Could you check a few things on this model? Use its own coordinates, in mm. Face numbers are marked on the shaded views. A direction names the side the tool comes from. Give positions to 0.01 mm unless a question says otherwise; leave off trailing zeros. Order: outer loops, then holes, each group sorted by start corner. A loop starts at its lowest first (then second) coordinate and runs counter-clockwise, first axis right, second up. Notation, with made-up numbers: M 73,23.5 L 114,23.5 A13 ccw 114,32.5 Z; hole C 55,72.5 d10. An arc over 180 degrees is marked long. Use a Markdown table: item, result. Add a question column.
```python
from build123d import *

# Parameters (mm, degrees)
BOSS_EXTRUDE1_DEPTH      = 50.8
BOSS_EXTRUDE1_DEPTH_BACK = 8.89
SKETCH3_W                = 168.91
SKETCH3_H                = 143.51
SKETCH3_W_2              = 148.59
SKETCH3_H_2              = 123.19
SKETCH3_3_W              = 148.59
SKETCH3_3_H              = 123.19
BOSS_EXTRUDE2_DEPTH      = 8.89
BOSS_EXTRUDE3_DEPTH      = 59.69
CUT_EXTRUDE1_DEPTH       = 239.691156361
CUT_EXTRUDE1_DEPTH_BACK  = 239.691156361
SKETCH5_R                = 4.445
SKETCH5_R_2              = 1.000000032
SKETCH5_R_3              = 1
FILLET1_R                = 5.08
SKETCH7_W                = 88.9
SKETCH7_H                = 95.25
BOSS_EXTRUDE4_DEPTH      = 12.7
CHAMFER1_SIZE            = 21.336
CHAMFER2_START           = -153
CHAMFER2_OUTLINE_W       = 18
CHAMFER2_OUTLINE_H       = 17
CHAMFER2_DEPTH           = 6.894626535
CHAMFER3_START           = -186
CHAMFER3_OUTLINE_W       = 15
CHAMFER3_OUTLINE_H       = 17
CHAMFER3_DEPTH           = 6.430939091
CHAMFER4_SIZE            = 5.08
CHAMFER5_SIZE            = 5.08
FILLET3_R                = 10.16
CHAMFER6_SIZE            = 5.08
CUT_EXTRUDE2_DEPTH       = 275.484237722
CUT_EXTRUDE2_DEPTH_BACK  = 275.484237722
SKETCH8_R                = 5.08
SKETCH9_R                = 2
SKETCH9_R_2              = 2.000000064
CUT_EXTRUDE3_DEPTH       = 12.7
SKETCH10_W               = 12.7
SKETCH10_H               = 43.18
BOSS_EXTRUDE5_DEPTH      = 50.8
SKETCH11_W               = 27.305
SKETCH11_H               = 50.8
CUT_EXTRUDE4_DEPTH       = 12.7
FILLET4_R                = 5.08
SKETCH12_R               = 15.875
CUT_EXTRUDE5_DEPTH       = 2.032
CUT_EXTRUDE6_START       = -2.032
SKETCH13_R               = 15.875
CUT_EXTRUDE6_DEPTH       = 2.032
FILLET5_R                = 5.08
FILLET6_R                = 5.08
SKETCH15_R               = 7.62
CUT_EXTRUDE7_DEPTH       = 5.08
BOSS_EXTRUDE6_DEPTH      = 12.7
FILLET9_R                = 6.35
BOSS_EXTRUDE7_START      = -12.7
BOSS_EXTRUDE7_DEPTH      = 12.7


with BuildPart() as part:
    # Sketch3 → Boss-Extrude1 (new, two sides: drawn at the far end of the back side and taken through both)
    with BuildSketch(Plane(origin=(0, 0, 0), x_dir=(1, 0, 0), z_dir=(0, 1, 0)).offset(-BOSS_EXTRUDE1_DEPTH_BACK)):
        Rectangle(SKETCH3_W, SKETCH3_H)
        Rectangle(SKETCH3_W_2, SKETCH3_H_2, mode=Mode.SUBTRACT)
    extrude(amount=BOSS_EXTRUDE1_DEPTH + BOSS_EXTRUDE1_DEPTH_BACK)

    # Sketch3<3> → Boss-Extrude2 (add)
    with BuildSketch(Plane(origin=(0, 0, 0), x_dir=(1, 0, 0), z_dir=(0, 1, 0))):
        Rectangle(SKETCH3_3_W, SKETCH3_3_H)
    extrude(amount=-BOSS_EXTRUDE2_DEPTH)

    # Sketch4 → Boss-Extrude3 (add)
    with BuildSketch(Plane(origin=(0, -8.89, 0), x_dir=(-1, 0, 0), z_dir=(0, -1, 0))):
        Polygon((137.454999918, 60.325), (84.455, 60.325), (84.455, 43.815), (126.024999918, 43.815), (126.024999918, 23.495), (137.454999918, 23.495), align=None)
        Polygon((126.025, -43.815), (84.455, -43.815), (84.455, -60.325), (137.455, -60.325), (137.455, -23.495), (126.025, -23.495), align=None)
        Polygon((-84.455, 43.815), (-84.455, 60.325), (-137.454999918, 60.325), (-137.454999918, 23.495), (-126.024999918, 23.495), (-126.024999918, 43.815), align=None)
        Polygon((-84.455, -43.815), (-126.025, -43.815), (-126.025, -23.495), (-137.455, -23.495), (-137.455, -60.325), (-84.455, -60.325), align=None)
    extrude(amount=-BOSS_EXTRUDE3_DEPTH)

    # Sketch5 → Cut-Extrude1 (cut, two sides: drawn at the far end of the back side and taken through both)
    with BuildSketch(Plane.ZY.offset(84.455).offset(-CUT_EXTRUDE1_DEPTH_BACK)):
        with Locations(Location((0, 20.955, 0), (0, 0, 180))):
            Circle(SKETCH5_R)
        with Locations(Location((-9.017, 20.955, 0), (0, 0, 180))):
            Circle(SKETCH5_R_2)
        with Locations(Location((9.017, 20.955, 0), (0, 0, 180))):
            Circle(SKETCH5_R_3)
        with Locations(Location((0.017538483, 29.972, 0), (0, 0, 180))):
            Circle(SKETCH5_R_3)
        with Locations(Location((-0.055629344, 11.938, 0), (0, 0, 180))):
            Circle(SKETCH5_R_3)
    extrude(amount=CUT_EXTRUDE1_DEPTH + CUT_EXTRUDE1_DEPTH_BACK, mode=Mode.SUBTRACT)

    # Fillet1
    fillet1_edges = [part.edges().sort_by_distance(p)[0] for p in [
        (84.455, 20.955, -60.325),
        (84.455, 20.955, -43.815),
        (-84.455, 20.955, -43.815),
        (-84.455, 20.955, -60.325),
        (-84.455, 20.955, 43.815),
        (-84.455, 20.955, 60.325),
        (84.455, 20.955, 71.755),
        (-84.455, 20.955, 71.755),
        (84.455, 20.955, 60.325),
        (84.455, 20.955, 43.815),
    ]]
    fillet(fillet1_edges, radius=FILLET1_R)

    # Sketch7 → Boss-Extrude4 (add)
    with BuildSketch(Plane.ZY.offset(84.455)):
        with Locations((-116.205, 28.287736962)):
            Rectangle(SKETCH7_W, SKETCH7_H)
    extrude(amount=-BOSS_EXTRUDE4_DEPTH)

    # Chamfer1
    # the kernel refuses this chamfer: 21.336 mm, written as the material it takes off along each edge
    with BuildSketch(Plane(origin=(-139.324428231, 75.912736962, -71.755), x_dir=(0, -1, 0), z_dir=(1, 0, 0))) as chamfer1_piece_1:
        Polygon((CHAMFER1_SIZE, 0), (0, CHAMFER1_SIZE), (0, 0), align=None)
    extrude(amount=122.438856462, mode=Mode.SUBTRACT)
    with BuildSketch(Plane(origin=(-139.324428231, -19.337263038, -71.755), x_dir=(0, 1, 0), z_dir=(1, 0, 0))) as chamfer1_piece_2_section:
        Polygon((CHAMFER1_SIZE, 0), (0, -CHAMFER1_SIZE), (0, 0), align=None)
    chamfer1_piece_2 = extrude(amount=122.438856462, mode=Mode.PRIVATE)
    chamfer1_piece_2 = split(chamfer1_piece_2, bisect_by=Plane(origin=(-139.324428231, -8.89, -71.755), z_dir=(0, -1, 0)), keep=Keep.TOP, mode=Mode.PRIVATE)
    add(chamfer1_piece_2, mode=Mode.SUBTRACT)

    # Chamfer2: read off the stored shape, not the designer's step
    # Chamfer2 outline → Chamfer2 (cut)
    with BuildSketch(Plane(origin=(0, 0, 0), x_dir=(0.8737038499063027, -0.34397789366389886, -0.34397789366389886), z_dir=(0.4864582023760161, 0.6178019170175401, 0.6178019170175401)).offset(CHAMFER2_START)):
        with Locations((-8, 99.5)):
            Rectangle(CHAMFER2_OUTLINE_W, CHAMFER2_OUTLINE_H)
    extrude(amount=CHAMFER2_DEPTH, mode=Mode.SUBTRACT)

    # Chamfer3: read off the stored shape, not the designer's step
    # Chamfer3 outline → Chamfer3 (cut)
    with BuildSketch(Plane(origin=(0, 0, 0), x_dir=(0.8164965809277258, 0.40824829046386313, -0.40824829046386313), z_dir=(0.5773502691896258, -0.5773502691896258, 0.5773502691896258)).offset(CHAMFER3_START)):
        with Locations((29.5, -59.5)):
            Rectangle(CHAMFER3_OUTLINE_W, CHAMFER3_OUTLINE_H)
    extrude(amount=CHAMFER3_DEPTH, mode=Mode.SUBTRACT)

    # Chamfer4
    chamfer4_edges = [part.edges().sort_by_distance(p)[0] for p in [
        (-74.295, 25.4, 61.595),
        (74.295, 25.4, 61.595),
    ]]
    chamfer(chamfer4_edges, length=CHAMFER4_SIZE)

    # Chamfer5
    chamfer5_edges = [part.edges().sort_by_distance(p)[0] for p in [
        (6.35, 50.8, -71.755),
    ]]
    chamfer(chamfer5_edges, length=CHAMFER5_SIZE)

    # Fillet3
    fillet3_edges = [part.edges().sort_by_distance(p)[0] for p in [
        (-71.755, 18.415, -71.755),
    ]]
    fillet(fillet3_edges, radius=FILLET3_R)

    # Chamfer6
    chamfer6_edges = [part.edges().sort_by_distance(p)[0] for p in [
        (-78.105, 75.912736962, -93.091),
    ]]
    chamfer(chamfer6_edges, length=CHAMFER6_SIZE)

    # Mirror1: part across plane


with BuildPart() as part_1:
    add(part.part)
    add(part.part.mirror(Plane.ZY))

    # Sketch8 → Cut-Extrude2 (cut, two sides: drawn at the far end of the back side and taken through both)
    with BuildSketch(Plane(origin=(-71.755, 0, 0), x_dir=(0, 0, -1), z_dir=(1, 0, 0)).offset(-CUT_EXTRUDE2_DEPTH_BACK)):
        with Locations((140.97, 37.812736962)):
            Circle(SKETCH8_R)
    extrude(amount=CUT_EXTRUDE2_DEPTH + CUT_EXTRUDE2_DEPTH_BACK, mode=Mode.SUBTRACT)

    # Sketch9 → Cut-Extrude3 (cut)
    with BuildSketch(Plane(origin=(0, 50.8, 0), x_dir=(1, 0, 0), z_dir=(0, 1, 0))):
        with Locations(Location((-78.769563039, 66.590491676, 0), (0, 0, 270))):
            Circle(SKETCH9_R)
        with Locations(Location((-79.531563039, 33.026568856, 0), (0, 0, 270))):
            Circle(SKETCH9_R)
        with Locations(Location((-78.642563039, -62.223431144, 0), (0, 0, 270))):
            Circle(SKETCH9_R_2)
        with Locations(Location((78.595485178, -62.865, 0), (0, 0, 270))):
            Circle(SKETCH9_R)
        with Locations(Location((78.595485178, 66.675, 0), (0, 0, 270))):
            Circle(SKETCH9_R)
        with Locations(Location((81.135485178, 32.385, 0), (0, 0, 270))):
            Circle(SKETCH9_R)
    extrude(amount=-CUT_EXTRUDE3_DEPTH, mode=Mode.SUBTRACT)

    # Sketch10 → Boss-Extrude5 (add)
    with BuildSketch(Plane(origin=(0, 0, 0), x_dir=(1, 0, 0), z_dir=(0, 1, 0))):
        with Locations((-25.7556, 40.005)):
            Rectangle(SKETCH10_W, SKETCH10_H)
    extrude(amount=BOSS_EXTRUDE5_DEPTH)

    # Sketch11 → Cut-Extrude4 (cut)
    with BuildSketch(Plane.XY.offset(-61.595)):
        with Locations((-58.1025, 25.4)):
            Rectangle(SKETCH11_W, SKETCH11_H)
    extrude(amount=-CUT_EXTRUDE4_DEPTH, mode=Mode.SUBTRACT)

    # Fillet4
    # the kernel refuses this fillet: 5.08 mm, written as the material it takes off along each edge
    with BuildSketch(Plane(origin=(-44.45, 58.42, -71.755), x_dir=(1, 0, 0), z_dir=(0, -1, 0))) as fillet4_piece_1:
        with BuildLine():
            CenterArc((FILLET4_R, FILLET4_R), FILLET4_R, 180, 90)
            Line((0, FILLET4_R), (-FILLET4_R * 0.02, FILLET4_R))
            Line((-FILLET4_R * 0.02, FILLET4_R), (-FILLET4_R * 0.02, -FILLET4_R * 0.02))
            Line((-FILLET4_R * 0.02, -FILLET4_R * 0.02), (FILLET4_R, -FILLET4_R * 0.02))
            Line((FILLET4_R, -FILLET4_R * 0.02), (FILLET4_R, 0))
        make_face()
    extrude(amount=58.42, mode=Mode.SUBTRACT)
    with BuildSketch(Plane(origin=(-44.45, 0, -61.595), x_dir=(0, 0, -1), z_dir=(0, 1, 0))) as fillet4_piece_2:
        with BuildLine():
            CenterArc((FILLET4_R, -FILLET4_R), FILLET4_R, 90, 90)
            Line((0, -FILLET4_R), (-FILLET4_R * 0.02, -FILLET4_R))
            Line((-FILLET4_R * 0.02, -FILLET4_R), (-FILLET4_R * 0.02, FILLET4_R * 0.02))
            Line((-FILLET4_R * 0.02, FILLET4_R * 0.02), (FILLET4_R, FILLET4_R * 0.02))
            Line((FILLET4_R, FILLET4_R * 0.02), (FILLET4_R, 0))
        make_face()
    extrude(amount=63.5, mode=Mode.SUBTRACT)
    with BuildSketch(Plane(origin=(-71.755, 61.798522628, -61.595), x_dir=(0, 0, -1), z_dir=(0, -1, 0))) as fillet4_piece_3:
        with BuildLine():
            CenterArc((4.399409051, -5.08), FILLET4_R, 90, 60)
            Line((0, -2.54), (-0.087988181, -2.4892))
            ThreePointArc((-0.087988181, -2.4892), (-0.1016, -1.27), (-0.1016, 0))
            Line((-0.1016, 0), (0, 0.1016))
            Line((0, 0.1016), (4.399409051, 0.1016))
            Line((4.399409051, 0.1016), (4.399409051, 0))
        make_face()
    extrude(amount=61.798522628, mode=Mode.SUBTRACT)

    # Sketch12 → Cut-Extrude5 (cut)
    with BuildSketch(Plane(origin=(-74.295, 0, 0), x_dir=(0, 0, -1), z_dir=(1, 0, 0))):
        with Locations((0, 20.955)):
            Circle(SKETCH12_R)
    extrude(amount=-CUT_EXTRUDE5_DEPTH, mode=Mode.SUBTRACT)

    # Sketch13 → Cut-Extrude6 (cut)
    with BuildSketch(Plane.ZY.offset(-74.295).offset(CUT_EXTRUDE6_START)):
        with Locations(Location((0, 20.955, 0), (0, 0, 180))):
            Circle(SKETCH13_R)
    extrude(amount=CUT_EXTRUDE6_DEPTH, mode=Mode.SUBTRACT)

    # Fillet5
    fillet5_edges = [part_1.edges().sort_by_distance(p)[0] for p in [
        (-19.4056, 0, -40.005),
        (-19.4056, 25.4, -61.595),
        (-32.1056, 25.4, -61.595),
        (-32.1056, 0, -40.005),
        (-25.7556, 0, -18.415),
    ]]
    fillet(fillet5_edges, radius=FILLET5_R)

    # Fillet6
    fillet6_edges = [part_1.edges().sort_by_distance(p)[0] for p in [
        (-71.755, -19.337263038, -126.873),
        (-84.455, -19.337263038, -121.873),
        (84.455, -19.337263038, -121.873),
        (71.755, -19.337263038, -126.873),
    ]]
    fillet(fillet6_edges, radius=FILLET6_R)

    # Sketch15 → Cut-Extrude7 (cut)
    with BuildSketch(Plane.ZY.offset(32.1056)):
        with Locations((-41.275, 27.94)):
            Circle(SKETCH15_R)
    extrude(amount=-CUT_EXTRUDE7_DEPTH, mode=Mode.SUBTRACT)

    # Sketch17 → Boss-Extrude6 (add)
    with BuildSketch(Plane.ZY.offset(84.455)):
        with BuildLine():
            Line((-150.655, 75.912736962), (-98.171, 75.912736962))
            ThreePointArc((-98.171, 75.912736962), (-104.299654898, 91.920369087), (-115.471784879, 104.91991557))
            ThreePointArc((-115.471784879, 104.91991557), (-120.708410024, 105.664070641), (-123.768126586, 101.349659413))
            ThreePointArc((-123.768126586, 101.349659413), (-132.250831328, 83.387695455), (-150.655, 75.912736962))
        make_face()
    extrude(amount=-BOSS_EXTRUDE6_DEPTH)

    # Fillet9
    fillet9_edges = [part_1.edges().sort_by_distance(p)[0] for p in [
        (-137.455, 20.955, 60.325),
        (137.455, 20.955, 60.325),
    ]]
    fillet(fillet9_edges, radius=FILLET9_R)

    # Sketch18 → Boss-Extrude7 (add)
    with BuildSketch(Plane(origin=(84.455, 0, 0), x_dir=(0, 0, -1), z_dir=(1, 0, 0)).offset(BOSS_EXTRUDE7_START)):
        with BuildLine():
            ThreePointArc((123.768126586, 101.349659413), (132.250831328, 83.387695455), (150.655, 75.912736962))
            Line((150.655, 75.912736962), (98.171, 75.912736962))
            ThreePointArc((98.171, 75.912736962), (104.299654898, 91.920369087), (115.471784879, 104.91991557))
            ThreePointArc((115.471784879, 104.91991557), (120.708410024, 105.664070641), (123.768126586, 101.349659413))
        make_face()
    extrude(amount=BOSS_EXTRUDE7_DEPTH)


solid = part_1.part
```
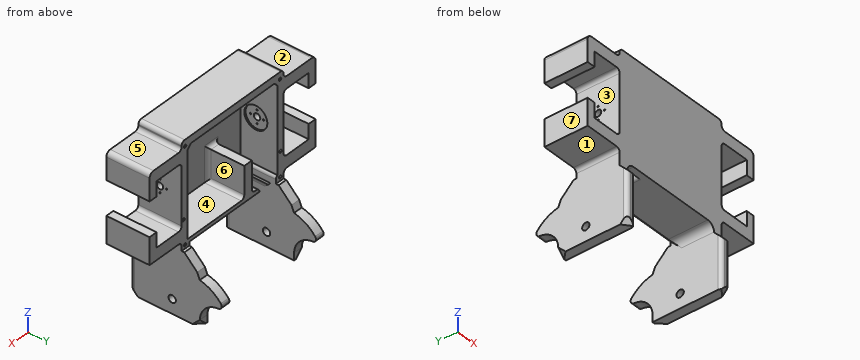
1) Suppose I cut it at B-B on z = -140.97. Please give me the cut outline in (x, y) (3 decimals), and give its area (3 significant figures).
2) For the marked faces 1, 2, 3 and 4, which set-ups out of +Z, -Z, +X, -X, +Y, -Y let a thin tool reach every point of the face, with its end or its side?
3) For pin 1 (12 mm diameter, centred on y = 52.5, z = 47, fed in from -X) (3 decimals); pin 2 (1 mm diameter, centred on y = 7.5, z = 66, fed in from -X) (3 decimals); pin 3 (4.5 mm diameter, centred on x = -78.64, z = 62.22, fed in from -Y); pin 4 (5.5 mm diameter, centred on x = -134, y = 30, fed in from +Z), each with a flat end and sliding along its axis, tell me the tip position at first contact or that it passes through.
4) Please list where these lines run through material, in increasing order: line 1 (X direction, y = -7, z = -33.5) (3 decimals); line 2 (Z direction, x = 108, y = 40) (3 decimals); line 3 (X direction, y = 27.5, z = -139) (3 decimals). Write a range as from..to.
5) We'd pull the mould along Z, two halves only. Please class the marked faces 5, 6 and 7: pulls with the +Z half, pulls with the -Z half, needs draft (parallel to the pull), parting line crosses it, or undercut.
6) Suppose I cut it at C-C on x = 26.5. Please give me the cut outline in (y, z) (3 decimals), and give its area (3 significant figures).
7) Suppose I cut it at A-A on x = 109.5. Please give me the cut outline in (y, z) (3 decimals), and give its area (3 significant figures).
Values found:
| question | item | result |
|---|---|---|
| 1 | outline | M -84.455,-14.257 A5.08 ccw -79.375,-19.337 L -76.835,-19.337 A5.08 ccw -71.755,-14.257 L -71.755,32.733 L -84.455,32.733 Z; M -84.455,42.893 L -71.755,42.893 L -71.755,77.831 L -84.455,77.831 Z; M 71.755,-14.257 A5.08 ccw 76.835,-19.337 L 79.375,-19.337 A5.08 ccw 84.455,-14.257 L 84.455,32.733 L 71.755,32.733 Z; M 71.755,42.893 L 84.455,42.893 L 84.455,77.831 L 71.755,77.831 Z |
| 1 | area | 2,190 mm^2 |
| 2 | face 1 | -Z, -X, +Y, -Y |
| 2 | face 2 | +Z, -X, +Y, -Y |
| 2 | face 3 | +Y, -Y |
| 2 | face 4 | +Y |
| 3 | pin 1 | stops at x = -137.455 |
| 3 | pin 2 | stops at x = -84.455 |
| 3 | pin 3 | stops at y = -8.89 |
| 3 | pin 4 | stops at z = 60.32 |
| 4 | line 1 | x = -137.455..-126.025, -84.455..84.455, 126.025..137.455 |
| 4 | line 2 | z = -60.325..-43.815, 43.815..60.325 |
| 4 | line 3 | x = -84.455..-71.755, 71.755..84.455 |
| 5 | face 5 | pulls with the +Z half |
| 5 | face 6 | undercut |
| 5 | face 7 | needs draft |
| 6 | outline | M -8.89,-71.755 L 45.72,-71.755 L 50.8,-66.675 L 50.8,-61.595 L 0,-61.595 L 0,61.595 L 50.8,61.595 L 50.8,71.755 L -8.89,71.755 Z |
| 6 | area | 2,300 mm^2 |
| 7 | outline | M -8.89,-60.325 L 50.8,-60.325 L 50.8,-43.815 L -8.89,-43.815 Z; M -8.89,43.815 L 50.8,43.815 L 50.8,60.325 L -8.89,60.325 Z |
| 7 | area | 1,970 mm^2 |
